For this review, take the finished solid that the model builds, in its own axes (mm). Give positions to 0.01 mm unless a question says otherwise; leave off trailing zeros. Loops run counter-clockwise (first coordinate to the right, second up) from the corner with the lowest first, then second, coordinate; pieces in that order, holes last.
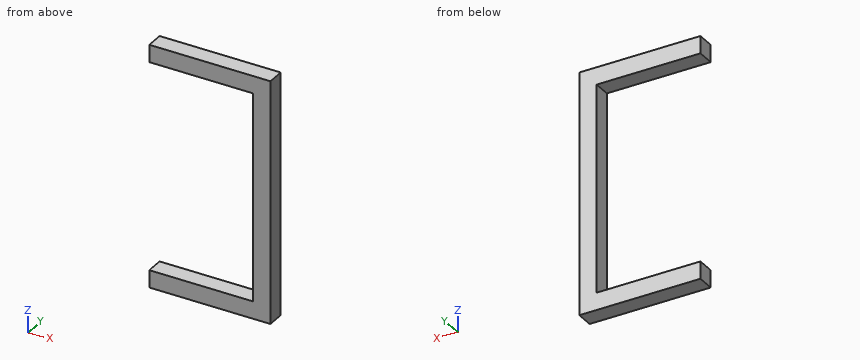
```python
from build123d import *

# Parameters (mm, degrees)
BOX244_W     = 12
BOX244_H     = 2
BOX244_DEPTH = 2
BOX245_W     = 12
BOX245_H     = 2
BOX245_DEPTH = 2
BOX243_W     = 2
BOX243_H     = 2
BOX243_DEPTH = 28


with BuildPart() as cube232:
    # Box244 → Box244 (new body)
    with BuildSketch(Plane(origin=(96.5, 53, -8.5), x_dir=(1, 0, 0), z_dir=(0, 0, 1))):
        with Locations((6, 1)):
            Rectangle(BOX244_W, BOX244_H)
    extrude(amount=BOX244_DEPTH)


with BuildPart() as cube233:
    # Box245 → Box245 (new body)
    with BuildSketch(Plane(origin=(96.5, 53, -34.5), x_dir=(1, 0, 0), z_dir=(0, 0, 1))):
        with Locations((6, 1)):
            Rectangle(BOX245_W, BOX245_H)
    extrude(amount=BOX245_DEPTH)


with BuildPart() as fusion077:
    # Box243 → Box243 (new body)
    with BuildSketch(Plane(origin=(108.5, 53, -34.5), x_dir=(1, 0, 0), z_dir=(0, 0, 1))):
        with Locations((1, 1)):
            Rectangle(BOX243_W, BOX243_H)
    extrude(amount=BOX243_DEPTH)

    # Fusion077: union Cube232, Cube233
    add(cube232.part)
    add(cube233.part)


solid = fusion077.part
```
Item 1: Take a section at B-B on y = 53.3. Give the boundary of the cut face in (x, z), and give its area (3 significant figures).
Answer:
outline: (96.5, -34.5) - (110.5, -34.5) - (110.5, -6.5) - (96.5, -6.5) - (96.5, -8.5) - (108.5, -8.5) - (108.5, -32.5) - (96.5, -32.5) - close
area: 104 mm2
Item 2: Take a section at C-C on z = -10. Give the boundary of the cut face in (x, y).
Answer:
outline: (108.5, 53) - (110.5, 53) - (110.5, 55) - (108.5, 55) - close
Item 3: For L1, parallel to Z at x = 102.75, y = 54.55; L2, parallel to X at y = 53.6, z = -31, list the stretches that pass through material, from the lowest coordinate up.
Answer:
L1: z = -34.5 to -32.5, -8.5 to -6.5
L2: x = 108.5 to 110.5
Item 4: Take a section at A-A on x = 107.25. Give the boundary of the cut face in (y, z).
Answer:
outline: (53, -34.5) - (55, -34.5) - (55, -32.5) - (53, -32.5) - close; (53, -8.5) - (55, -8.5) - (55, -6.5) - (53, -6.5) - close
